The drawing under review shows one solid part. Ordinate dimensions are in mm from its lowest x, y, z. Give positions to 0.01 mm unless a question says otherwise; leave off trailing zeros. Write each loop counter-clockwise with the first axis right and the second up, starting at its lowest first coordinate (ties: lowest second). Pieces come first, ordered by that corner, then holes.
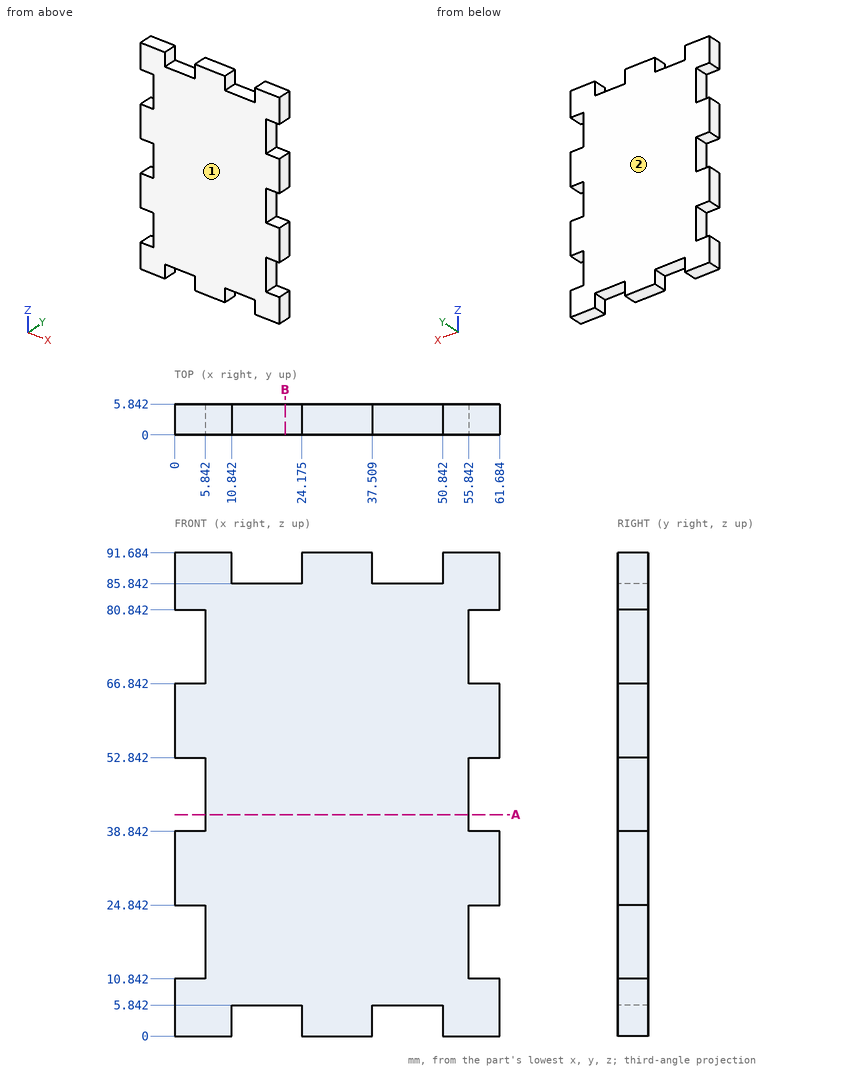
1) To check wall thickness, follow probe 1 along X at (y, z) = (3.15, 5.5) (1 decimal); probe 2 along X at (y, z) = (2.3, 45); probe 3 along Z at (x, y) = (39, 1.35). State the ranges of each line that lie inside material, in increasing order.
2) The part is to be moulded in two halves that separate along Y. For the marked faces 1 and 2, say which applies: +Y half, -Y half, draft (parallel to the pull), parting line (faces both ways), or undercut.
3) Insertion check: pin 1 (2 mm diameter, centred on x = 45, y = 2.5, fed in from -Z); pin 2 (1.8 mm diameter, centred on y = 2, z = 73, fed in from +X); pin 3 (3 mm diameter, centred on y = 1.5, z = 75, fed in from -X). Each pin has a flat end and moves straight along its axis. Give the tip position at first contact, or say it passes through.
4) Consider section B-B, the plane x = 21. Give the boundary of the cut face in (y, z), then the cut area to 3 significant figures.
5) Consider section A-A, the plane z = 42. Give the boundary of the cut face in (x, y).
Answer block:
1. probe 1: x = 0 to 10.8, 24.2 to 37.5, 50.8 to 61.7
1. probe 2: x = 5.84 to 55.84
1. probe 3: z = 5.84 to 85.84
2. face 1: -Y half
2. face 2: +Y half
3. pin 1: stops at z = 5.84
3. pin 2: stops at x = 55.84
3. pin 3: stops at x = 5.84
4. outline: (0, 5.84) - (5.84, 5.84) - (5.84, 85.84) - (0, 85.84) - close
4. area: 467 mm2
5. outline: (5.84, 0) - (55.84, 0) - (55.84, 5.84) - (5.84, 5.84) - close
